Geometry: final body of the model. Coordinates: model frame, mm. A direction names the side the tool comes from. Give positions to 0.01 mm unless a question says otherwise; leave off trailing zeros. Write each loop counter-clockwise with the first axis right and the second up, starting at its lowest first coordinate (ties: lowest second). Pieces come first, ordered by that corner, then holes. Notation, with made-up numbers: M 8.25,32 L 36.25,32 A21 cw 36.25,53 Z; hole C 33,28.25 d4. An arc over 180 degrees is marked long. Answer as a JSON object with one key per item and string values.
from build123d import *

# Parameters (mm, degrees)
F0_W     = 50.8
F0_H     = 101.6
F1_DEPTH = 850.9
F2_W     = 50.8
F2_H     = 101.6
F2_W_2   = 25.4
F2_H_2   = 44.45
F3_DEPTH = 50.8
F4_W     = 25.4
F4_H     = 44.45
F5_DEPTH = 50.801


# Not quite as in the source:
# - a pattern or mirror of a feature is missing from the dataset's text; its kind, count and spacing are read off the source's solid


with BuildPart() as f1:
    # F0 (on Right) → F1 (new body, symmetric)
    with BuildSketch(Plane.YZ):
        Rectangle(F0_W, F0_H)
    extrude(amount=F1_DEPTH, both=True)

    # F2 (on face) → F3 (cut)
    with BuildSketch(Plane(origin=(-850.9, 0, 0), x_dir=(0, -1, 0), z_dir=(-1, 0, 0))):
        Rectangle(F2_W, F2_H)
        Rectangle(F2_W_2, F2_H_2, mode=Mode.SUBTRACT)
    f3 = extrude(amount=-F3_DEPTH, mode=Mode.SUBTRACT)

    # F3_copies: F3 across plane
    add(f3.mirror(Plane(origin=(0, 0, 0), x_dir=(0, 0, 1), z_dir=(1, 0, 0))), mode=Mode.SUBTRACT)

    # F4 (on face) → F5 (cut, through all)
    with BuildSketch(Plane.XZ.offset(25.4)):
        with Locations((-762, 0)):
            Rectangle(F4_W, F4_H)
        with Locations((-254, 0)):
            Rectangle(F4_W, F4_H)
    f5 = extrude(amount=-F5_DEPTH, mode=Mode.SUBTRACT)

    # F5_copies: F5 across plane
    add(f5.mirror(Plane(origin=(0, 0, 0), x_dir=(0, 0, 1), z_dir=(1, 0, 0))), mode=Mode.SUBTRACT)


solid = f1.part
1) Line query: line 1 (X direction, y = 9, z = -18); line 2 (X direction, y = -22.5, z = -0.5); line 3 (Z direction, x = 754, y = 7) (3 decimals). Output: solid intervals per line, ascending. Write a range as from..to.
Geometry check:
{"line 1": "x = -850.9..-774.7, -749.3..-266.7, -241.3..241.3, 266.7..749.3, 774.7..850.9", "line 2": "x = -800.1..-774.7, -749.3..-266.7, -241.3..241.3, 266.7..749.3, 774.7..800.1", "line 3": "z = -50.8..-22.225, 22.225..50.8"}
2) Set-up query: faces 1 (the flat face through (-826, 12.7, 0)), 2 (the flat face through (-826, -12.7, 0)), 3 (the flat face through (241.3, 0, 0)), 4 (the flat face through (826, 12.7, 0)). Return all of +Z, -Z, +X, -X, +Y, -Y with unobstructed straight access to the full face (end or side cutting, diameter ignored); none if empty.
Geometry check:
{"face 1": "+Z, -Z, -X, +Y", "face 2": "+Z, -Z, -X, -Y", "face 3": "+Y, -Y", "face 4": "+Z, -Z, +X, +Y"}
3) Contact query for flat-ended pins moving along their axis: P1, Ø22, axis at x = -817, z = 5, coming from the -Y side; P2, Ø2, axis at y = 12, z = -35.5, coming from the +X side; P3, Ø20.5, axis at x = -814.5, y = -0.5, coming from the -Z side (3 decimals). Output: stop coordinate, or through.
Geometry check:
{"P1": "stops at y = -12.7", "P2": "stops at x = 800.1", "P3": "stops at z = -22.225"}
4) Cut plane A-A on z = -4. Return loops of the section in (x, y), and give its area (3 significant figures).
Geometry check:
{"outline": "M -850.9,-12.7 L -800.1,-12.7 L -800.1,-25.4 L -774.7,-25.4 L -774.7,25.4 L -800.1,25.4 L -800.1,12.7 L -850.9,12.7 Z; M -749.3,-25.4 L -266.7,-25.4 L -266.7,25.4 L -749.3,25.4 Z; M -241.3,-25.4 L 241.3,-25.4 L 241.3,25.4 L -241.3,25.4 Z; M 266.7,-25.4 L 749.3,-25.4 L 749.3,25.4 L 266.7,25.4 Z; M 774.7,-25.4 L 800.1,-25.4 L 800.1,-12.7 L 850.9,-12.7 L 850.9,12.7 L 800.1,12.7 L 800.1,25.4 L 774.7,25.4 Z", "area": "78,700 mm2"}
5) Cut plane B-B on y = 5. Return loops of the section in (x, z) (3 decimals).
Geometry check:
{"outline": "M -850.9,-22.225 L -800.1,-22.225 L -800.1,-50.8 L 800.1,-50.8 L 800.1,-22.225 L 850.9,-22.225 L 850.9,22.225 L 800.1,22.225 L 800.1,50.8 L -800.1,50.8 L -800.1,22.225 L -850.9,22.225 Z; hole M -774.7,-22.225 L -749.3,-22.225 L -749.3,22.225 L -774.7,22.225 Z; hole M -266.7,-22.225 L -241.3,-22.225 L -241.3,22.225 L -266.7,22.225 Z; hole M 241.3,-22.225 L 266.7,-22.225 L 266.7,22.225 L 241.3,22.225 Z; hole M 749.3,-22.225 L 774.7,-22.225 L 774.7,22.225 L 749.3,22.225 Z"}
6) Pull-direction query (Z, two-part tool) for faces 5 (the flat face through (11, 0, 50.8)), 6 (the flat face through (826, -12.7, 0)), 7 (the flat face through (-774.7, 0, 0)), 8 (the flat face through (-749.3, 0, 0)); classes: pulls with the +Z half, pulls with the -Z half, needs draft (parallel to the pull), parting line crosses it, or undercut.
Geometry check:
{"face 5": "pulls with the +Z half", "face 6": "needs draft", "face 7": "undercut", "face 8": "undercut"}
